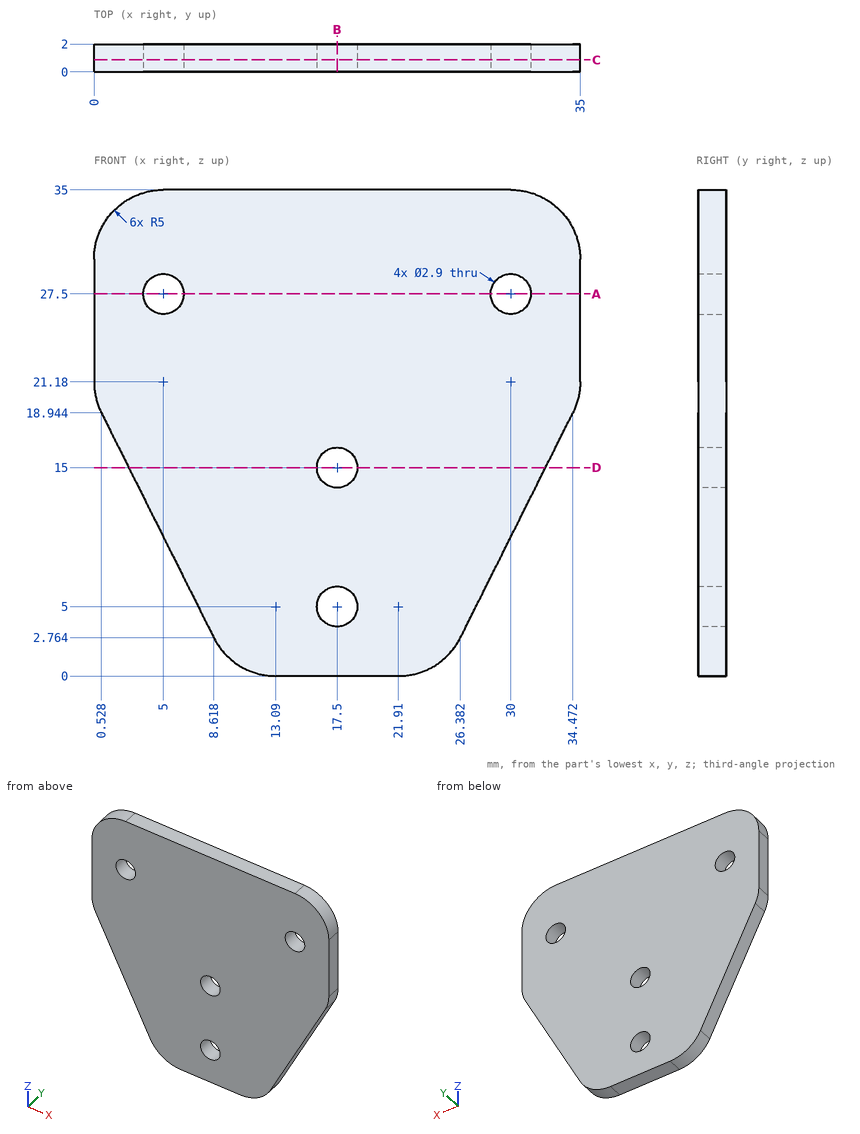
Input: dimensioned drawing with shaded views. Units: mm. Origin: part minimum x, y, z. Coordinates: 2 decimals unless noted, no trailing zeros. Write each loop counter-clockwise with the first axis right and the second up, starting at its lowest first coordinate (ties: lowest second). Pieces come first, ordered by that corner, then holes. Notation, with made-up numbers: M 61.5,33 L 99.5,33 A18 cw 99.5,38 Z; hole C 56.25,-27 d11. An arc over 180 degrees is marked long. Answer as a JSON object with one key per item and string values. Group by question number.
(1) Section B-B on x = 17.5. Output: boundary loops of the cut face in (y, z), plus the area to 3 significant figures.
(2) Section C-C on y = 0.85. Output: boundary loops of the cut face in (x, z).
(3) Section D-D on z = 15. Output: boundary loops of the cut face in (x, y), plus the area to 3 significant figures.
(4) Ray query, line 1 along Z through (x, y) = (18, 1.25); line 2 along Z through (x, y) = (5, 1.25); line 3 along X through (y, z) = (1.35, 5). Return the intervals inside material, ascending. Write a range as [from, to].
(5) Section A-A on z = 27.5. Output: boundary loops of the cut face in (x, y), plus the area to 3 significant figures.
(6) Contact query for flat-ended pins moving along their axis: P1, Ø3.5, axis at x = 17.5, z = 5, coming from the -Y side; P2, Ø2.5, axis at x = 17.5, z = 15, coming from the -Y side. Output: stop coordinate, or through.
Result set:
{
 "1": {"outline": "M 0,0 L 2,0 L 2,3.55 L 0,3.55 Z; M 0,6.45 L 2,6.45 L 2,13.55 L 0,13.55 Z; M 0,16.45 L 2,16.45 L 2,35 L 0,35 Z", "area": "58.4 mm2"},
 "2": {"outline": "M 0,21.18 A5 ccw 0.53,18.94 L 8.62,2.76 A5 ccw 13.09,0 L 21.91,0 A5 ccw 26.38,2.76 L 34.47,18.94 A5 ccw 35,21.18 L 35,30 A5 ccw 30,35 L 5,35 A5 ccw 0,30 Z; hole C 5,27.5 d2.9; hole C 17.5,5 d2.9; hole C 17.5,15 d2.9; hole C 30,27.5 d2.9"},
 "3": {"outline": "M 2.5,0 L 16.05,0 L 16.05,2 L 2.5,2 Z; M 18.95,0 L 32.5,0 L 32.5,2 L 18.95,2 Z", "area": "54.2 mm2"},
 "4": {"line 1": "z = [0, 3.64], [6.36, 13.64], [16.36, 35]", "line 2": "z = [10, 26.05], [28.95, 35]", "line 3": "x = [7.5, 16.05], [18.95, 27.5]"},
 "5": {"outline": "M 0,0 L 3.55,0 L 3.55,2 L 0,2 Z; M 6.45,0 L 28.55,0 L 28.55,2 L 6.45,2 Z; M 31.45,0 L 35,0 L 35,2 L 31.45,2 Z", "area": "58.4 mm2"},
 "6": {"P1": "stops at y = 0", "P2": "passes through"}
}
